Work out the finished part from the listing and answer in its coordinate system (mm). Face numbers are marked on the shaded views. A direction names the side the tool comes from. Coordinates: 2 decimals unless noted, no trailing zeros. Order: outer loops, then holes, each group sorted by start corner. A loop starts at its lowest first (then second) coordinate and runs counter-clockwise, first axis right, second up. Notation, with made-up numbers: M 62.25,-1.5 L 93.25,-1.5 A18 ccw 93.25,26.5 Z; hole C 55,69.25 d8. An arc over 180 degrees is marked long. Use a Markdown table: item, result.
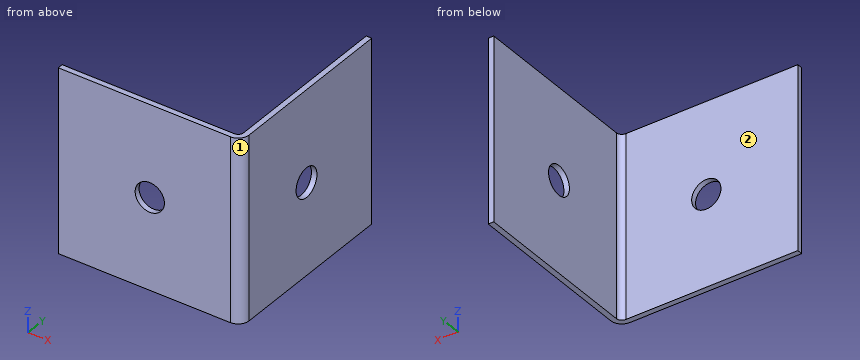
from build123d import *

# Parameters (mm, degrees)
SKETCH1_W              = 25.4
SKETCH1_H              = 25.4
SKETCH1_R              = 2.032
BOSS_EXTRUDE1_DEPTH    = 0.762
SKETCH2_W              = 25.4
SKETCH2_H              = 25.4
SKETCH2_R              = 2.032
BOSS_EXTRUDE2_DEPTH    = 0.762
CONVERT_SOLID1_START   = -12.7
CONVERT_SOLID1_DEPTH   = 25.4
CONVERT_SOLID1_2_DEPTH = 25.4


# Read off the part's stored shape, not the designer's step: Convert-Solid1
with BuildPart() as part:
    # Sketch1 → Boss-Extrude1 (new body)
    with BuildSketch(Plane(origin=(0, 0, 0), x_dir=(1, 0, 0), z_dir=(0, 1, 0))):
        Rectangle(SKETCH1_W, SKETCH1_H)
        with Locations(Location((0, 0, 0), (0, 0, 90))):
            Circle(SKETCH1_R, mode=Mode.SUBTRACT)
    extrude(amount=BOSS_EXTRUDE1_DEPTH)

    # Sketch2 → Boss-Extrude2 (add)
    with BuildSketch(Plane(origin=(12.7, 0, 0), x_dir=(0, 0, -1), z_dir=(1, 0, 0))):
        with Locations((0, 12.7)):
            Rectangle(SKETCH2_W, SKETCH2_H)
        with Locations((0, 12.7)):
            Circle(SKETCH2_R, mode=Mode.SUBTRACT)
    extrude(amount=-BOSS_EXTRUDE2_DEPTH)

    # Convert-Solid1 outline → Convert-Solid1 (cut)
    with BuildSketch(Plane.XY.offset(CONVERT_SOLID1_START)):
        with BuildLine():
            Line((12.7, 0), (12.7, 1.524))
            ThreePointArc((12.7, 1.524), (12.253630735, 0.446369265), (11.176, 0))
            Line((11.176, 0), (12.7, 0))
        make_face()
    extrude(amount=CONVERT_SOLID1_DEPTH, mode=Mode.SUBTRACT)

    # Convert-Solid1 2 outline → Convert-Solid1 2 (add)
    with BuildSketch(Plane.XY.offset(CONVERT_SOLID1_START)):
        with BuildLine():
            Line((11.938, 0.762), (11.938, 1.524))
            ThreePointArc((11.938, 1.524), (11.714815367, 0.985184633), (11.176, 0.762))
            Line((11.176, 0.762), (11.938, 0.762))
        make_face()
    extrude(amount=CONVERT_SOLID1_2_DEPTH)


solid = part.part
1. Find the intervals of material crossed by probe 1 along X at (y, z) = (19.25, 10); probe 2 along Y at (x, z) = (-9.5, 10.75); probe 3 along Y at (x, z) = (12.25, 0), in increasing order.
Answers below:
| item | result |
|---|---|
| probe 1 | 11.94 to 12.7 |
| probe 2 | 0 to 0.76 |
| probe 3 | 0.44 to 10.67, 14.73 to 25.4 |
2. For the marked faces 1 and 2, determine the directions among +Z, -Z, +X, -X, +Y, -Y from which every point of the face is accessible in a straight line to the end or side of a thin tool.
Answers below:
| item | result |
|---|---|
| face 1 | +Z, -Z, +X, -Y |
| face 2 | +Z, -Z, -X, +Y |
3. Section D-D on z = -7 is taken. Determine the outline of the cut face in (x, y).
Answers below:
| item | result |
|---|---|
| outline | M -12.7,0 L 11.18,0 A1.52 ccw 12.7,1.52 L 12.7,25.4 L 11.94,25.4 L 11.94,1.52 A0.76 cw 11.18,0.76 L -12.7,0.76 Z |
4. Section B-B on x = 0 is taken. Determine the outline of the cut face in (y, z), then the cut area to 3 significant figures.
Answers below:
| item | result |
|---|---|
| outline | M 0,-12.7 L 0.76,-12.7 L 0.76,-2.03 L 0,-2.03 Z; M 0,2.03 L 0.76,2.03 L 0.76,12.7 L 0,12.7 Z |
| area | 16.3 mm² |
5. Section C-C on z = 0 is taken. Determine the outline of the cut face in (x, y), then the cut area to 3 significant figures.
Answers below:
| item | result |
|---|---|
| outline | M -12.7,0 L -2.03,0 L -2.03,0.76 L -12.7,0.76 Z; M 2.03,0 L 11.18,0 A1.52 ccw 12.7,1.52 L 12.7,10.67 L 11.94,10.67 L 11.94,1.52 A0.76 cw 11.18,0.76 L 2.03,0.76 Z; M 11.94,14.73 L 12.7,14.73 L 12.7,25.4 L 11.94,25.4 Z |
| area | 31.6 mm² |
6. Flat-ended cylindrical pins translate along their axes: P1, Ø5, axis at y = 11, z = 4.5, coming from the -X side; P2, Ø4, axis at x = 9, y = 22, coming from the -Z side; P3, Ø1.5, axis at x = -1.5, z = 2.5, coming from the +Y side. Find the tip coordinate at first contact, or state that the pin passes through.
Answers below:
| item | result |
|---|---|
| P1 | x = 11.94 |
| P2 | through |
| P3 | y = 0.76 |
7. Section A-A on y = 12.7 is taken. Determine the outline of the cut face in (x, z), then the cut area to 3 significant figures.
Answers below:
| item | result |
|---|---|
| outline | M 11.94,-12.7 L 12.7,-12.7 L 12.7,-2.03 L 11.94,-2.03 Z; M 11.94,2.03 L 12.7,2.03 L 12.7,12.7 L 11.94,12.7 Z |
| area | 16.3 mm² |
